Geometry check sheet. Reference: drawing and pictorial views, mm from the part's lowest x, y, z. A direction names the side the tool comes from. Coordinates: 2 decimals unless noted, no trailing zeros. Loops run counter-clockwise (first coordinate to the right, second up) from the corner with the lowest first, then second, coordinate; pieces in that order, holes last. Notation, with made-up numbers: (-28, 68) -> (-11, 68) arc R12 cw to (-11, 85) -> close; hole circle Ø7 at (42.25, 15). An arc over 180 degrees is marked (long way). Use CSV: the item, a comma, the result in double quotes.
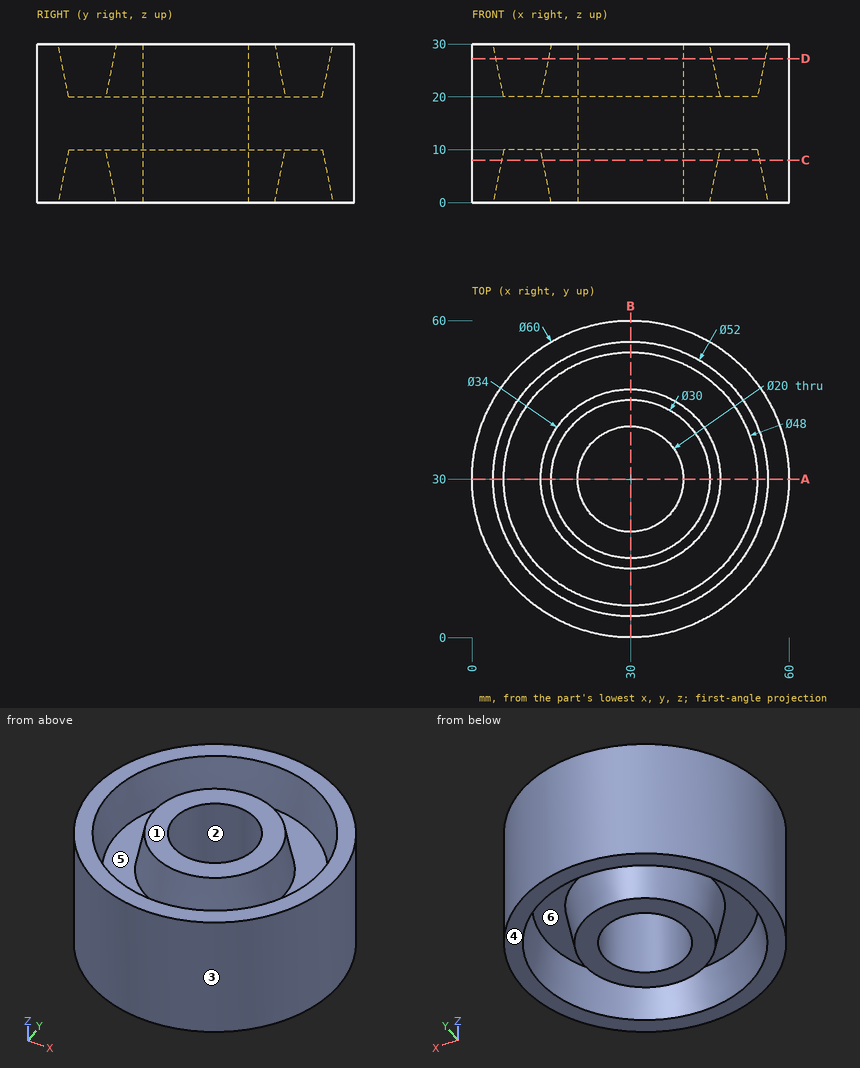
1) Thickness scan on line 1 along Y through (x, z) = (30, 10.75); line 2 along Y through (x, z) = (37.5, 24.75); line 3 along X through (y, z) = (31, 26). Record the ranges inside material, lowest first. Write a range as from..to.
Answer below:
line 1,"y = 0..20, 40..60"
line 2,"y = 0.95..6.2, 15.81..23.39, 36.61..44.19, 53.8..59.05"
line 3,"x = 0.02..4.82, 14.23..20.05, 39.95..45.77, 55.18..59.98"
2) Access from +Z, -Z, +X, -X, +Y, -Y to the whole of each face (thin tool, end or side, straight path). Record for the marked faces 4, 5 and 6.
Answer below:
face 4,"-Z, +X, -X, +Y, -Y"
face 5,"+Z"
face 6,"-Z"
3) Cross-section at C-C on z = 8. Record the boundary of the cut face in (x, y), and give its area (3 significant figures).
Answer below:
outline,"circle Ø60 at (30, 30); circle Ø33.2 at (30, 30); hole circle Ø48.8 at (30, 30); hole circle Ø20 at (30, 30)"
area,"1,510 mm²"
4) Cross-section at A-A on y = 30. Record the boundary of the cut face in (x, z).
Answer below:
outline,"(0, 0) -> (4, 0) -> (6, 10) -> (13, 10) -> (15, 0) -> (20, 0) -> (20, 30) -> (15, 30) -> (13, 20) -> (6, 20) -> (4, 30) -> (0, 30) -> close; (40, 0) -> (45, 0) -> (47, 10) -> (54, 10) -> (56, 0) -> (60, 0) -> (60, 30) -> (56, 30) -> (54, 20) -> (47, 20) -> (45, 30) -> (40, 30) -> close"
5) Cross-section at D-D on z = 27.25. Record the boundary of the cut face in (x, y), and give its area (3 significant figures).
Answer below:
outline,"circle Ø60 at (30, 30); circle Ø31.1 at (30, 30); hole circle Ø50.9 at (30, 30); hole circle Ø20 at (30, 30)"
area,"1,240 mm²"
6) Go/stop test with flat-tipped pins: pin 1 Ø4 at (y, z) = (13.5, 7.5) entering from -X; pin 2 Ø2 at (y, z) = (50.5, 7.5) entering from -X; pin 3 Ø4 at (y, z) = (43, 11) entering from -X. Record where each tip stops, or that it passes through.
Answer below:
pin 1,"stops at x = 3.74"
pin 2,"stops at x = 7.2"
pin 3,"stops at x = 2.09"
7) Draft check along X on the marked faces 1, 2 and 3. Enter one of: released by +X, released by -X, zero draft, split by the parting line, or undercut.
Answer below:
face 1,"zero draft"
face 2,"undercut"
face 3,"split by the parting line"
